Geometry: final body of the model. Coordinates: model frame, mm. A direction names the side the tool comes from. Coordinates: 2 decimals unless noted, no trailing zeros. Loops run counter-clockwise (first coordinate to the right, second up) from the corner with the lowest first, then second, coordinate; pieces in that order, holes last. Notation, with made-up numbers: (71, -32.75) - (100, -32.75) arc R15 cw to (100, -24.75) - close; hole circle Ø5 at (15.5, 58.5). An arc over 180 degrees is marked (long way). Put each result on its own line as item: value. Start each with the question number.
1) Section A-A on z = 9.25. Output: boundary loops of the cut face in (x, y).
2) Material intervals for line 1 along X through (y, z) = (93.5, 8.25); line 2 along Y through (x, z) = (70, 8.7); line 3 along Y through (x, z) = (70, 6.4), sorted ascending. Write a range as from..to.
3) Reachability of faces 1 (the flat face through (70, 137.4, 11)), 2 (the flat face through (83, 107, 10)), 3 (the flat face through (70, 98, 10.2)) from +Z, -Z, +X, -X, +Y, -Y: full face, straight path, thin tool, end or side. Return the list, or none.
4) Draft query along X for faces 4 (the flat face through (85, 108, 11)), 5 (the flat face through (70, 135.4, 10)), 6 (the cylindrical face through (56.804, 135.689, 11.141)), 7 (the flat face through (57, 108, 10)). Return one class per face: +X half, -X half, draft (parallel to the pull), parting line (faces both ways), or undercut.
5) Section C-C on x = 70. Output: boundary loops of the cut face in (y, z).
6) Section B-B on y = 98.4. Output: boundary loops of the cut face in (x, z), and give its area (3 significant figures).
7) Contact query for flat-ended pins moving along their axis: pin 1 Ø9 at (x, y) = (65, 120) entering from -Z; pin 2 Ø0.7 at (x, y) = (69.5, 98.5) entering from -Z. Output: stop coordinate, or through.
8) Section D-D on y = 109. Output: boundary loops of the cut face in (x, z), and give its area (3 significant figures).
```python
from build123d import *

# Parameters (mm, degrees)
PAD016_DEPTH    = 5.8
POCKET020_DEPTH = 3.8
SKETCH068_R     = 4
PAD017_DEPTH    = 6.8
SKETCH069_R     = 1.2
POCKET021_DEPTH = 5
FILLET002_R     = 2


with BuildPart() as part:
    # Sketch066 (on DatumPlane) → Pad016 (new body)
    with BuildSketch(Plane.XY.offset(14)):
        with BuildLine():
            Line((61, 137.4), (79, 137.4))
            ThreePointArc((85, 131.4), (83.242641, 135.642641), (79, 137.4))
            Line((85, 131.4), (85, 83.6))
            Line((85, 83.6), (55, 83.6))
            Line((55, 83.6), (55, 131.4))
            ThreePointArc((61, 137.4), (56.757359, 135.642641), (55, 131.4))
        make_face()
    extrude(amount=-PAD016_DEPTH)

    # Sketch067 (on Face8 of Pad016) → Pocket020 (cut)
    with BuildSketch(Plane(origin=(0, 0, 8.2), x_dir=(1, 0, 0), z_dir=(0, 0, -1))):
        with BuildLine():
            Line((57, -83.6), (83, -83.6))
            Line((83, -83.6), (83, -131.4))
            ThreePointArc((79, -135.4), (81.828427, -134.228427), (83, -131.4))
            Line((79, -135.4), (61, -135.4))
            ThreePointArc((57, -131.4), (58.171573, -134.228427), (61, -135.4))
            Line((57, -131.4), (57, -83.6))
        make_face()
    extrude(amount=-POCKET020_DEPTH, mode=Mode.SUBTRACT)

    # Sketch068 (on Face14 of Pocket020) → Pad017 (join)
    with BuildSketch(Plane(origin=(0, 0, 12), x_dir=(1, 0, 0), z_dir=(0, 0, -1))):
        with Locations((70, -98.4)):
            Circle(SKETCH068_R)
    extrude(amount=PAD017_DEPTH)

    # Sketch069 (on Face16 of Pad017) → Pocket021 (cut)
    with BuildSketch(Plane(origin=(0, 0, 5.2), x_dir=(1, 0, 0), z_dir=(0, 0, -1))):
        with Locations((70, -98.4)):
            Circle(SKETCH069_R)
    extrude(amount=-POCKET021_DEPTH, mode=Mode.SUBTRACT)

    # Fillet002
    fillet002_edges = [part.edges().sort_by_distance(p)[0] for p in [
        (66, 98.4, 12),
    ]]
    fillet(fillet002_edges, radius=FILLET002_R)


solid = part.part
```
Answer block:
1. outline: (55, 83.6) - (57, 83.6) - (57, 131.4) arc R4 cw to (61, 135.4) - (79, 135.4) arc R4 cw to (83, 131.4) - (83, 83.6) - (85, 83.6) - (85, 131.4) arc R6 ccw to (79, 137.4) - (61, 137.4) arc R6 ccw to (55, 131.4) - close; circle Ø8 at (70, 98.4); hole circle Ø2.4 at (70, 98.4)
2. line 1: x = 55..57, 83..85
2. line 2: y = 94.4..97.2, 99.6..102.4, 135.4..137.4
2. line 3: y = 94.4..97.2, 99.6..102.4
3. face 1: +Z, -Z, +X, -X, +Y
3. face 2: -Z, -Y
3. face 3: -Z
4. face 4: +X half
4. face 5: undercut
4. face 6: -X half
4. face 7: undercut
5. outline: (83.6, 12) - (92.4, 12) arc R2 cw to (94.4, 10) - (94.4, 5.2) - (97.2, 5.2) - (97.2, 10.2) - (99.6, 10.2) - (99.6, 5.2) - (102.4, 5.2) - (102.4, 10) arc R2 cw to (104.4, 12) - (135.4, 12) - (135.4, 8.2) - (137.4, 8.2) - (137.4, 14) - (83.6, 14) - close
6. outline: (55, 8.2) - (57, 8.2) - (57, 12) - (64, 12) arc R2 cw to (66, 10) - (66, 5.2) - (68.8, 5.2) - (68.8, 10.2) - (71.2, 10.2) - (71.2, 5.2) - (74, 5.2) - (74, 10) arc R2 cw to (76, 12) - (83, 12) - (83, 8.2) - (85, 8.2) - (85, 14) - (55, 14) - close
6. area: 119 mm²
7. pin 1: stops at z = 12
7. pin 2: stops at z = 10.2
8. outline: (55, 8.2) - (57, 8.2) - (57, 12) - (83, 12) - (83, 8.2) - (85, 8.2) - (85, 14) - (55, 14) - close
8. area: 75.2 mm²
